Read the model definition and answer for the solid it produces. Units are mm, in the model's axes. Face numbers are marked on the shaded views. A direction names the side the tool comes from. Coordinates: 2 decimals unless noted, no trailing zeros. Loops run counter-clockwise (first coordinate to the right, second up) from the corner with the lowest first, then second, coordinate; pieces in that order, holes last. Notation, with made-up numbers: (87, 26.25) -> (131, 26.25) arc R20 cw to (131, 35.25) -> close; hole circle Ø2 at (75.25, 87). An arc over 180 degrees is marked (long way). Answer as a JSON object with one key per item and string values. Group by question number.
Q1. The part is cut by section C-C on x = 2.2. Write down the section's boundary in (y, z), and give its area (3 significant figures).
Q2. For the marked faces 1, 2 and 3, determine the directions among +Z, -Z, +X, -X, +Y, -Y from which every point of the face is accessible in a straight line to the end or side of a thin tool.
Q3. The part is cut by section A-A on y = 0. Write down the section's boundary in (x, z).
Q4. Straight lines are drawn through the part: line 1 along Y through (x, z) = (1.65, 0); line 2 along X through (y, z) = (2, -2.5); line 3 along X through (y, z) = (4.75, 0). For each, find the intervals that lie inside material, in ascending order. Write a range as [from, to].
Q5. Determine the mould class of the marked faces 4, 5 and 6 for opening direction Y: released by +Y, released by -Y, zero draft, split by the parting line, or undercut.
Q6. The part is cut by section B-B on z = 0. Write down the section's boundary in (x, y), and give its area (3 significant figures).
Q7. This flat-tipped pin is pushed along its axis until it touches: P1, Ø4, axis at y = 0, z = 0, coming from the -X side. Where does it stop, or does it pass through?
Q8. The part is cut by section D-D on x = 1.3. Write down the section's boundary in (y, z), and give its area (3 significant figures).
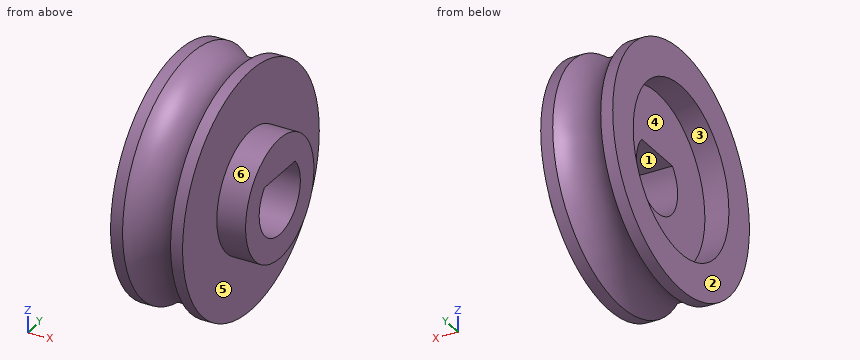
from build123d import *

# Parameters (mm, degrees)
SKETCH7_R               = 2.5
BOSS_EXTRUDE1_DEPTH     = 1.2
CUT_EXTRUDE1_DEPTH      = 2.2
CUT_EXTRUDE1_DEPTH_BACK = 4
SKETCH9_R               = 3.5
CUT_EXTRUDE2_DEPTH      = 1


with BuildPart() as part:
    # Sketch3 → Revolve1 (revolve)
    with BuildSketch(Plane.XY):
        with BuildLine():
            Line((-1.5, 0), (1.5, 0))
            Line((1.5, 0), (1.5, 5))
            Line((1.5, 5), (1, 5))
            ThreePointArc((1, 5), (0, 4.618033989), (-1, 5))
            Line((-1, 5), (-1.5, 5))
            Line((-1.5, 5), (-1.5, 0))
        make_face()
    revolve(axis=Axis((0, 0, 0), (1, 0, 0)))

    # Sketch7 → Boss-Extrude1 (add)
    with BuildSketch(Plane(origin=(1.5, 0, 0), x_dir=(0, 0, -1), z_dir=(1, 0, 0))):
        Circle(SKETCH7_R)
    extrude(amount=BOSS_EXTRUDE1_DEPTH)

    # Sketch5 → Cut-Extrude1 (cut, two sides)
    with BuildSketch(Plane(origin=(1.5, 0, 0), x_dir=(0, 0, -1), z_dir=(1, 0, 0))) as cut_extrude1_sk:
        with BuildLine():
            Line((-1, 1.125953933), (-1, -1.125953933))
            ThreePointArc((-1, -1.125953933), (1.505912434, 0), (-1, 1.125953933))
        make_face()
    extrude(amount=CUT_EXTRUDE1_DEPTH, mode=Mode.SUBTRACT)
    extrude(cut_extrude1_sk.sketch, amount=-CUT_EXTRUDE1_DEPTH_BACK, mode=Mode.SUBTRACT)

    # Sketch9 → Cut-Extrude2 (cut)
    with BuildSketch(Plane.ZY.offset(1.5)):
        Circle(SKETCH9_R)
    extrude(amount=-CUT_EXTRUDE2_DEPTH, mode=Mode.SUBTRACT)


solid = part.part
Final values:
{
 "1": {"outline": "circle Ø5 at (0, 0); hole (-1.13, 1) arc R1.51 ccw (long way) to (1.13, 1) -> close", "area": "13.3 mm2"},
 "2": {"face 1": "+X, -X", "face 2": "+Z, -Z, -X, +Y, -Y", "face 3": "-X"},
 "3": {"outline": "(-1.5, -5) -> (-1, -5) arc R1.5 cw to (1, -5) -> (1.5, -5) -> (1.5, -2.5) -> (2.7, -2.5) -> (2.7, -1.51) -> (-0.5, -1.51) -> (-0.5, -3.5) -> (-1.5, -3.5) -> close; (-1.5, 3.5) -> (-0.5, 3.5) -> (-0.5, 1) -> (2.7, 1) -> (2.7, 2.5) -> (1.5, 2.5) -> (1.5, 5) -> (1, 5) arc R1.5 cw to (-1, 5) -> (-1.5, 5) -> close"},
 "4": {"line 1": "y = [-2.5, -1.51], [1.51, 2.5]", "line 2": "x = [-0.5, 1.5]", "line 3": "x = [-1.5, -0.62], [0.62, 1.5]"},
 "5": {"face 4": "undercut", "face 5": "zero draft", "face 6": "split by the parting line"},
 "6": {"outline": "(-1.5, -5) -> (-1, -5) arc R1.5 cw to (1, -5) -> (1.5, -5) -> (1.5, -2.5) -> (2.7, -2.5) -> (2.7, -1.51) -> (-0.5, -1.51) -> (-0.5, -3.5) -> (-1.5, -3.5) -> close; (-1.5, 3.5) -> (-0.5, 3.5) -> (-0.5, 1.51) -> (2.7, 1.51) -> (2.7, 2.5) -> (1.5, 2.5) -> (1.5, 5) -> (1, 5) arc R1.5 cw to (-1, 5) -> (-1.5, 5) -> close", "area": "18.3 mm2"},
 "7": {"P1": "stops at x = -0.5"},
 "8": {"outline": "circle Ø10 at (0, 0); hole (-1.13, 1) arc R1.51 ccw (long way) to (1.13, 1) -> close", "area": "72.2 mm2"}
}
